CAD build for the part. Positions are in the model's coordinates, mm. Face numbers are marked on the shaded views. A direction names the side the tool comes from. Round coordinates to 2 decimals unless told otherwise and drop trailing zeros. Loops run counter-clockwise (first coordinate to the right, second up) from the corner with the lowest first, then second, coordinate; pieces in that order, holes last. Notation, with made-up numbers: M 7,-4 L 54,-4 A33 ccw 54,35 Z; hole C 77.5,39 d11. An arc over 180 degrees is marked long. Use a Markdown table: item, result. Add a question column.
(1) Band-saw the part on A-A, the plane y = 2.75. Write the cut outline in (x, z).
(2) Which spindle directions (+Z, -Z, +X, -X, +Y, -Y) get a long thin tool onto all of the face, cutting with end or side? Do the marked faces 1 and 2. Say none if no direction does.
(3) Band-saw the part on B-B, the plane x = 0. Write the cut outline in (y, z).
(4) Flat gauge pins, fed straight in: P1, Ø2, axis at x = 1, y = -3, coming from the +Z side; P2, Ø2, axis at y = 2.5, z = -6, coming from the -X side; P3, Ø3, axis at x = 4, z = -2, coming from the +Y side. Where does each tip first touch, or does it go through?
(5) Band-saw the part on D-D, the plane y = -0.75. Write the cut outline in (x, z).
(6) Band-saw the part on C-C, the plane z = -6.25. Write the cut outline in (x, y), and give its area (3 significant figures).
(7) Wall check: L1, parallel to Z at x = 0, y = 1.4; L2, parallel to Z at x = 0, y = 1.85; L3, parallel to Z at x = -0.75, y = -3.5. Give the ranges that are in metal, low to high.
(8) Two-plate mould, pull along X, no slides. Class the marked faces 3, 4 and 5: released by +X, released by -X, zero draft, split by the parting line, or undercut.
Autodesk Inventor part; units mm, degrees
ref_plane "Work Plane1" through (-5.6, 5.6, 0) normal (0, 1, 0) x (1, 0, 0)
ref_plane "YZ Plane" through (0, 0, 0) normal (1, 0, 0) x (0, 1, 0)
ref_plane "XZ Plane" through (0, 0, 0) normal (0, 1, 0) x (-1, 0, 0)
sketch "Sketch1" plane through (0, 0, 0) normal (0, 0, 1) x (1, 0, 0)
  circle A0 centre (0, 0) radius 5.6
  dimension "d0" = 11.2
extrude "Extrusion1" add sketch "Sketch1" against normal blind 9
ref_plane "Work Plane1" through (-5.6, 5.6, 0) normal (0, 1, 0) x (1, 0, 0)
sketch "Sketch3" plane through (-5.6, 5.6, 0) normal (0, 1, 0) x (1, 0, 0)
  circle A0 centre (5.6, 4.5) radius 1.2
  point P0 (5.6, 0)
  dimension "d9" = 2.4
hole "Hole1" at (0, 5.6, -4.5) direction (0, -1, 0) diameter 2.459 depth 5.6
sketch "Sketch4" plane through (0, 0, 0) normal (0, 0, 1) x (1, 0, 0)
  circle A0 centre (0, 0) radius 5.6
  circle A1 centre (0, 0) radius 1.75
  dimension "d17" = 3.5
extrude "Extrusion3" add sketch "Sketch4" along normal blind 6 contours A1
properties part number "gear motor"
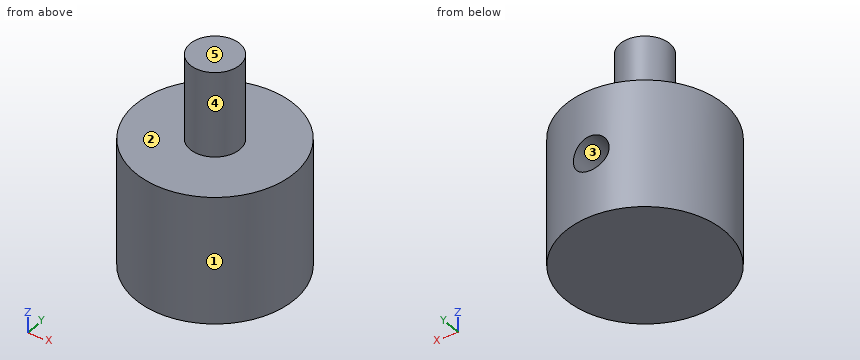
Return value:
| question | item | result |
|---|---|---|
| 1 | outline | M -4.88,-9 L 4.88,-9 L 4.88,0 L -4.88,0 Z; hole C 0,-4.5 d2.46 |
| 2 | face 1 | +Z, -Z |
| 2 | face 2 | +Z |
| 3 | outline | M -5.6,-9 L 5.6,-9 L 5.6,-5.73 L 0,-5.73 L 0,-3.27 L 5.6,-3.27 L 5.6,0 L 1.75,0 L 1.75,6 L -1.75,6 L -1.75,0 L -5.6,0 Z |
| 4 | P1 | z = 0 |
| 4 | P2 | x = -5.4 |
| 4 | P3 | y = 5.01 |
| 5 | outline | M -5.55,-9 L 5.55,-9 L 5.55,0 L 1.58,0 L 1.58,6 L -1.58,6 L -1.58,0 L -5.55,0 Z |
| 6 | outline | C 0,0 d11.2 |
| 6 | area | 98.5 mm^2 |
| 7 | L1 | -9 to -5.73, -3.27 to 6 |
| 7 | L2 | -9 to -5.73, -3.27 to 0 |
| 7 | L3 | -9 to 0 |
| 8 | face 3 | undercut |
| 8 | face 4 | split by the parting line |
| 8 | face 5 | zero draft |
